```python
from build123d import *

# Parameters (mm, degrees)
SKETCH1_R           = 22.5
BOSS_EXTRUDE1_DEPTH = 108.92387
SKETCH2_R           = 14.765011188
CUT_EXTRUDE1_DEPTH  = 114.476470935
CHAMFER1_SIZE       = 4.700246


with BuildPart() as part:
    # Sketch1 → Boss-Extrude1 (new body)
    with BuildSketch(Plane(origin=(0, 0, 0), x_dir=(1, 0, 0), z_dir=(0, 1, 0))):
        with Locations(Location((0, 0, 0), (0, 0, 270))):
            Circle(SKETCH1_R)
    extrude(amount=BOSS_EXTRUDE1_DEPTH)

    # Sketch2 → Cut-Extrude1 (cut, through all)
    with BuildSketch(Plane(origin=(0, 0, 0), x_dir=(1, 0, 0), z_dir=(0, 1, 0))):
        with Locations(Location((0, 0, 0), (0, 0, 270))):
            Circle(SKETCH2_R)
    extrude(amount=CUT_EXTRUDE1_DEPTH, mode=Mode.SUBTRACT)

    # Chamfer1
    chamfer1_edges = [part.edges().sort_by_distance(p)[0] for p in [
        (0, 0, -22.5),
        (0, 108.92387, -22.5),
    ]]
    chamfer(chamfer1_edges, length=CHAMFER1_SIZE)


solid = part.part
```
Model file for the job. Use its own axes, mm. Coordinates: 2 decimals unless noted, no trailing zeros. Order: outer loops, then holes, each group sorted by start corner. A loop starts at its lowest first (then second) coordinate and runs counter-clockwise, first axis right, second up. Notation, with made-up numbers: (35.25, 80.25) -> (66.25, 80.25) arc R34 cw to (66.25, 118.25) -> close; hole circle Ø6 at (60, 76.5). An arc over 180 degrees is marked (long way). Answer as a JSON object with one key per item and string values. Group by question number.
1) Pull direction Z, two halves, no side cores. Call faces 1 (the face through (-8.98, 53.7, -11.72)), 2 (the face through (-8.618, 53.765, 20.784)), 3 (the face through (15, 108.924, 3)): +Z half, -Z half, draft (parallel to the pull), parting line (faces both ways), or undercut.
2) Cut at A-A, the plane x = 0. Write the cut outline in (y, z), then the cut area to 3 significant figures.
3) Flat gauge pins, fed straight in: pin 1 (3 mm diameter, centred on y = 37.5, z = 3, fed in from -X); pin 2 (3 mm diameter, centred on y = 35.5, z = 14.5, fed in from -X); pin 3 (8 mm diameter, centred on x = -5, y = 29, fed in from -Z). Where does each tip first touch, or does it go through?
4) Cut at B-B, the plane z = 0. Write the cut outline in (x, y).
5) Cut at C-C, the plane y = 59. Write the cut outline in (x, z), then the cut area to 3 significant figures.
6) Drill centre lines: L1, parallel to X at y = 66, z = 0; L2, parallel to X at y = 7, z = 6; L3, parallel to Z at x = 8.5, y = 78. Where is each one in solid material? Low to high.
Check values:
{
 "1": {"face 1": "undercut", "face 2": "parting line", "face 3": "draft"},
 "2": {"outline": "(0, -17.8) -> (4.7, -22.5) -> (104.22, -22.5) -> (108.92, -17.8) -> (108.92, -14.77) -> (0, -14.77) -> close; (0, 14.77) -> (108.92, 14.77) -> (108.92, 17.8) -> (104.22, 22.5) -> (4.7, 22.5) -> (0, 17.8) -> close", "area": "1,640 mm²"},
 "3": {"pin 1": "stops at x = -22.45", "pin 2": "stops at x = -18.36", "pin 3": "stops at z = -22.48"},
 "4": {"outline": "(-22.5, 4.7) -> (-17.8, 0) -> (-14.77, 0) -> (-14.77, 108.92) -> (-17.8, 108.92) -> (-22.5, 104.22) -> close; (14.77, 0) -> (17.8, 0) -> (22.5, 4.7) -> (22.5, 104.22) -> (17.8, 108.92) -> (14.77, 108.92) -> close"},
 "5": {"outline": "circle Ø45 at (0, 0); hole circle Ø29.53 at (0, 0)", "area": "906 mm²"},
 "6": {"L1": "x = -22.5 to -14.77, 14.77 to 22.5", "L2": "x = -21.69 to -13.49, 13.49 to 21.69", "L3": "z = -20.83 to -12.07, 12.07 to 20.83"}
}
